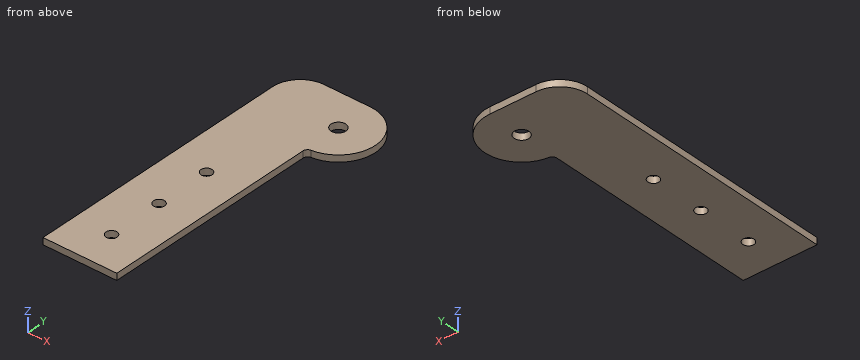
Autodesk Inventor part; units mm, degrees
ref_plane "YZ Plane" through (0, 0, 0) normal (1, 0, 0) x (0, 1, 0)
ref_plane "XZ Plane" through (0, 0, 0) normal (0, 1, 0) x (-1, 0, 0)
ref_plane "XY Plane" through (0, 0, 0) normal (0, 0, 1) x (1, 0, 0)
sketch "Sketch1" plane through (0, 0, 0) normal (0, 0, 1) x (1, 0, 0)
  line L0 (0, 0) -> (25.4, 0)
  line L1 (25.4, 0) -> (25.4, 101.6)
  line L2 (25.4, 101.6) -> (0, 101.6)
  line L3 (0, 101.6) -> (0, 0)
  arc A0 (25.4, 76.2) -> (25.4, 101.6) centre (25.4, 88.9) ccw
  dimension "d0" = 101.6
  dimension "d1" = 25.4
  dimension "d2" = 25.4
extrude "Extrusion1" add sketch "Sketch1" along normal blind 2.286
sketch "Sketch3" plane through (0, 0, 2.286) normal (0, 0, 1) x (1, 0, 0)
  line L0 (0, 101.6) -> (0, 0)
  line L1 (0, 0) -> (25.4, 0)
  line L2 (25.4, 101.6) -> (0, 101.6)
  line L3 (25.4, 0) -> (25.4, 76.2)
  line L4 (0, 0) -> (25.4, 0)
  line L5 (25.4, 0) -> (25.4, 63.5)
  line L6 (25.4, 63.5) -> (0, 63.5)
  line L7 (0, 63.5) -> (0, 0)
  point P0 (12.7, 50.8)
  point P1 (12.7, 12.7)
  point P2 (12.7, 31.75)
  point P3 (12.7, 0)
  dimension "d50" = 12.7
  dimension "d53" = 38.1
  dimension "d54" = 63.5
  dimension "d55" = 19.05
hole "Hole1" at (12.7, 50.8, 2.286) at (12.7, 12.7, 2.286) at (12.7, 31.75, 2.286) direction (0, 0, -1) diameter 3.81 end through all
sketch "Sketch4" plane through (0, 0, 2.286) normal (0, 0, 1) x (1, 0, 0)
  line L0 (25.4, 0) -> (25.4, 76.2)
  arc A0 (25.4, 76.2) -> (25.4, 101.6) centre (25.4, 88.9) ccw
  point P0 (0, 0)
hole "Hole2" at (25.4, 88.9, 2.286) direction (0, 0, -1) diameter 5.08 end through all
fillet "Fillet1" radius 9.525 1 edges at (0, 101.6, 1.143)
fillet "Fillet2" radius 1.5875 1 edges at (25.4, 76.2, 1.143)
equation "\"d2\" = d1"
properties part number "WJ_CLB_027_LifterBracket" material "Aluminum 6061"
Design review of the part built by this model. Coordinates are the model's own, in mm. Give positions to 0.01 mm unless a question says otherwise; leave off trailing zeros. Write each loop counter-clockwise with the first axis right and the second up, starting at its lowest first coordinate (ties: lowest second). Pieces come first, ordered by that corner, then holes. Notation, with made-up numbers: M 47.25,70.5 L 73.25,70.5 A22 ccw 73.25,93.5 Z; hole C 6.25,68.25 d7. An arc over 180 degrees is marked long. Answer as a JSON object with one key per item and string values. Group by question number.
1) For line 1 along Y through (x, z) = (12.7, 0.8) (3 decimals); line 2 along X through (y, z) = (50.8, 0.85) (3 decimals); line 3 along X through (y, z) = (88.9, 1.5), list the stretches that pass through material, from the lowest coordinate up.
2) We need section A-A (x = 12.7). Give the boundary of the cut face in (y, z) (3 decimals), and give its area (3 significant figures).
3) Clearance check with flat-ended pins moving along their axes: pin 1 Ø4.5 at (x, y) = (12.7, 50.8) entering from -Z; pin 2 Ø1.1 at (y, z) = (31.5, 1.5) entering from +X; pin 3 Ø2 at (x, y) = (31, 75.5) entering from +Z. State where each tip first meets the part, or that it passes through.
4) We need section B-B (y = 88.9). Give the boundary of the cut face in (x, z), and give its area (3 significant figures).
5) We need section D-D (y = 12.7). Give the boundary of the cut face in (x, z) (3 decimals), and give its area (3 significant figures).
6) We need section C-C (z = 1.15). Count the separate pieces of the cut face and the enclosed holes in it, and give its area (3 significant figures).
Answer key:
{
 "1": {"line 1": "y = 0 to 10.795, 14.605 to 29.845, 33.655 to 48.895, 52.705 to 101.6", "line 2": "x = 0 to 10.795, 14.605 to 25.4", "line 3": "x = 0 to 22.86, 27.94 to 38.1"},
 "2": {"outline": "M 0,0 L 10.795,0 L 10.795,2.286 L 0,2.286 Z; M 14.605,0 L 29.845,0 L 29.845,2.286 L 14.605,2.286 Z; M 33.655,0 L 48.895,0 L 48.895,2.286 L 33.655,2.286 Z; M 52.705,0 L 101.6,0 L 101.6,2.286 L 52.705,2.286 Z", "area": "206 mm²"},
 "3": {"pin 1": "stops at z = 0", "pin 2": "stops at x = 25.4", "pin 3": "passes through"},
 "4": {"outline": "M 0,0 L 22.86,0 L 22.86,2.29 L 0,2.29 Z; M 27.94,0 L 38.1,0 L 38.1,2.29 L 27.94,2.29 Z", "area": "75.5 mm²"},
 "5": {"outline": "M 0,0 L 10.795,0 L 10.795,2.286 L 0,2.286 Z; M 14.605,0 L 25.4,0 L 25.4,2.286 L 14.605,2.286 Z", "area": "49.4 mm²"},
 "6": {"separate pieces": "1", "enclosed holes": "4", "area": "2,760 mm²"}
}
